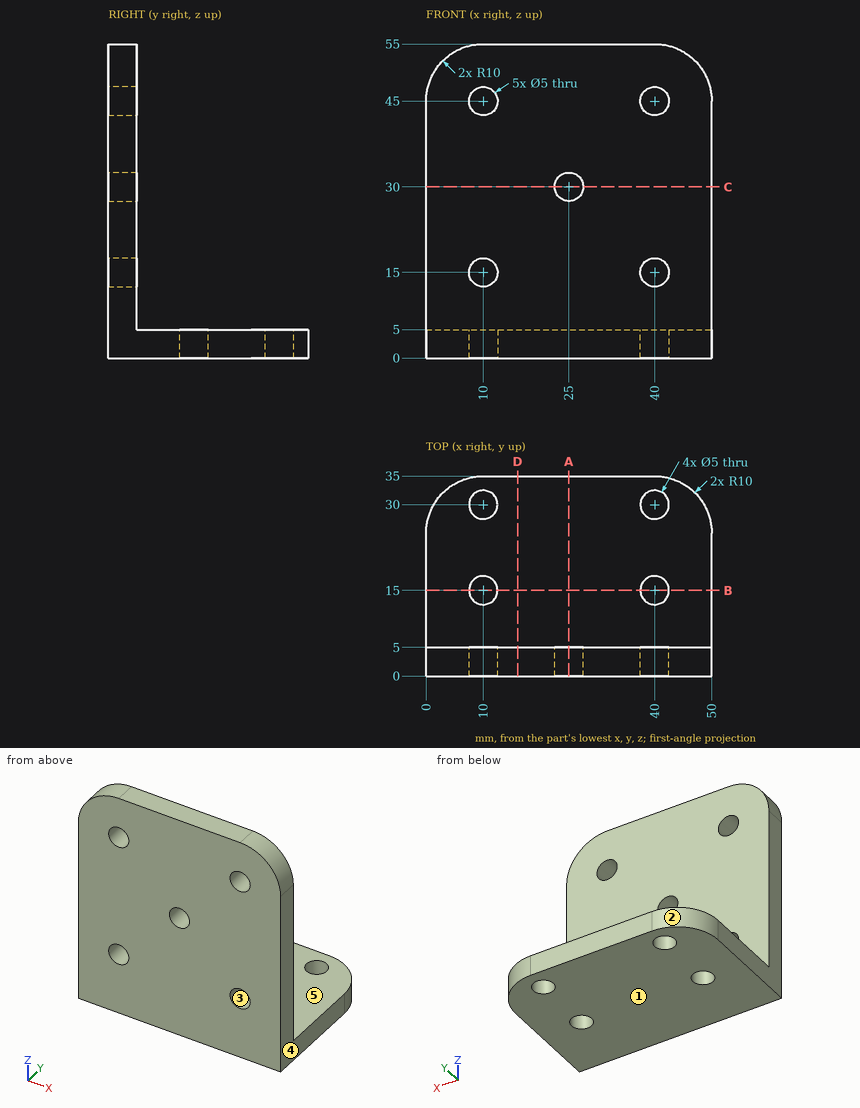
Input: dimensioned drawing with shaded views. Units: mm. Origin: part minimum x, y, z. A direction names the side the tool comes from. Coordinates: 2 decimals unless noted, no trailing zeros. Loops run counter-clockwise (first coordinate to the right, second up) from the corner with the lowest first, then second, coordinate; pieces in that order, holes last. Notation, with made-up numbers: M -25.75,-3 L 29.25,-3 A19 cw 29.25,14 Z; hole C 55.25,-35.5 d11. An arc over 180 degrees is marked long. One line per item, written item: value. Start each with the question number.
1) Cut plane D-D (x = 16). Return loops of the section in (y, z).
2) Draft query along X for the marked faces 1, 2 and 3. Return one class per face: released by +X, released by -X, zero draft, split by the parting line, or undercut.
3) Cut plane A-A (x = 25). Return loops of the section in (y, z), then the cut area to 3 significant figures.
4) Cut plane B-B (y = 15). Return loops of the section in (x, z).
5) Cut plane C-C (z = 30). Return loops of the section in (x, y), then the cut area to 3 significant figures.
6) Pin query (flat end, axial travel): P1, Ø10, axis at x = 44, z = 30, coming from the +Y side; P2, Ø6, axis at x = 40, y = 30, coming from the +Z side. Return the tip coordinate at first contact, or that it passes through.
7) Material intervals for L1, parallel to Y at x = 10, z = 1.2; L2, parallel to Y at x = 5.5, z = 18, sorted ascending. Write a range as from..to.
8) Reachability of the marked faces 4 and 5 from +Z, -Z, +X, -X, +Y, -Y: full face, straight path, thin tool, end or side. Return the list, or none.
Evaluation:
1. outline: M 0,0 L 35,0 L 35,5 L 5,5 L 5,55 L 0,55 Z
2. face 1: zero draft
2. face 2: released by -X
2. face 3: undercut
3. outline: M 0,0 L 35,0 L 35,5 L 5,5 L 5,27.5 L 0,27.5 Z; M 0,32.5 L 5,32.5 L 5,55 L 0,55 Z
3. area: 400 mm^2
4. outline: M 0,0 L 7.5,0 L 7.5,5 L 0,5 Z; M 12.5,0 L 37.5,0 L 37.5,5 L 12.5,5 Z; M 42.5,0 L 50,0 L 50,5 L 42.5,5 Z
5. outline: M 0,0 L 22.5,0 L 22.5,5 L 0,5 Z; M 27.5,0 L 50,0 L 50,5 L 27.5,5 Z
5. area: 225 mm^2
6. P1: y = 5
6. P2: z = 5
7. L1: 0..12.5, 17.5..27.5, 32.5..35
7. L2: 0..5
8. face 4: +Z, -Z, +X, +Y, -Y
8. face 5: +Z, +X, -X, +Y
